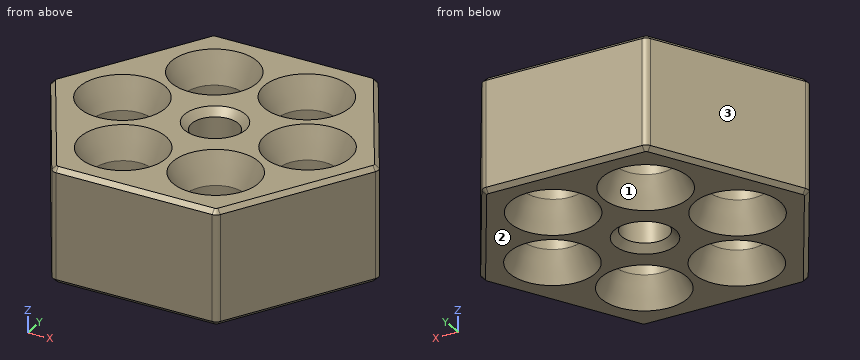
Autodesk Fusion 360 part; units mm, degrees
sketch "Sketch1" plane through (0, 0, 0) normal (0, 0, 1) x (1, 0, 0)
  line L0 (-5.7735, 10) -> (-11.547, 0)
  line L1 (-11.547, 0) -> (-5.7735, -10)
  line L2 (-5.7735, -10) -> (5.7735, -10)
  line L3 (5.7735, -10) -> (11.547, 0)
  line L4 (11.547, 0) -> (5.7735, 10)
  line L5 (5.7735, 10) -> (-5.7735, 10)
  circle A0 centre (0, 0) radius 1.625
  circle A1 centre (-3.25, 5.6292) radius 2.05
  line L6 (0, 0) -> (-5.7735, 10) construction
  circle A2 centre (-6.5, 0) radius 2.05
  circle A3 centre (-3.25, -5.6292) radius 2.05
  circle A4 centre (3.25, -5.6292) radius 2.05
  circle A5 centre (6.5, 0) radius 2.05
  circle A6 centre (3.25, 5.6292) radius 2.05
  circle A7 centre (0, 0) radius 6.5 construction
  dimension "d1" = 10
  dimension "d2" = 3.25
  dimension "d4" = 4.1
  dimension "d9" = 360
  dimension "d10" = 13
extrude "Extrude1" add sketch "Sketch1" along normal blind 8
chamfer "Chamfer3" distance 0.5 angle 45 1 edges at (-1.515, 0.5876, 0)
chamfer "Chamfer3" distance 0.5 angle 45 1 edges at (-1.515, 0.5876, 8)
fillet "Fillet1" radius 0.5 6 edges at (-5.7735, -10, 4) (5.7735, -10, 4) (11.547, 0, 4) (5.7735, 10, 4) (-5.7735, 10, 4) (-11.547, 0, 4)
chamfer "Chamfer4" distance 0.3 angle 45 24 edges at (0, -10, 8) (5.7348, -9.933, 8) (8.6603, -5, 8) (11.4697, 0, 8) (8.6603, 5, 8) (5.7348, 9.933, 8) (0, 10, 8) (-5.7348, 9.933, 8) (-8.6603, 5, 8) (-11.4697, 0, 8) (-8.6603, -5, 8) (-5.7348, -9.933, 8) (0, -10, 0) (5.7348, -9.933, 0) (8.6603, -5, 0) (11.4697, 0, 0) (8.6603, 5, 0) (5.7348, 9.933, 0) (0, 10, 0) (-5.7348, 9.933, 0) (-8.6603, 5, 0) (-11.4697, 0, 0) (-8.6603, -5, 0) (-5.7348, -9.933, 0)
chamfer "Chamfer2" distance 2 angle 25 6 edges at (1.3387, 6.3705, 8) (-5.1613, 6.3705, 8) (-8.4113, 0.7413, 8) (-5.1613, -4.8879, 8) (1.3387, -4.8879, 8) (4.5887, 0.7413, 8) measured on face at (5.2975, 5.527, 5.3333) measured on face at (-1.2025, 5.527, 5.3333) measured on face at (-4.4525, -0.1022, 5.3333) measured on face at (-1.2025, -5.7313, 5.3333) measured on face at (5.2975, -5.7313, 5.3333) measured on face at (8.5475, -0.1022, 5.3333)
chamfer "Chamfer5" distance 2 angle 25 6 edges at (-5.1613, -4.8879, 0) (1.3387, -4.8879, 0) (4.5887, 0.7413, 0) (1.3387, 6.3705, 0) (-5.1613, 6.3705, 0) (-8.4113, 0.7413, 0) measured on face at (-1.2102, -5.8333, 2) measured on face at (5.2898, -5.8333, 2) measured on face at (8.5398, -0.2041, 2) measured on face at (5.2898, 5.4251, 2) measured on face at (-1.2102, 5.4251, 2) measured on face at (-4.4602, -0.2041, 2)
CAD build for the part. Positions are in the model's coordinates, mm. Face numbers are marked on the shaded views. Round coordinates to 2 decimals unless told otherwise and drop trailing zeros. Write each loop counter-clockwise with the first axis right and the second up, starting at its lowest first coordinate (ties: lowest second). Pieces come first, ordered by that corner, then holes. Notation, with made-up numbers: (-19, 74.25) -> (35, 74.25) arc R24 ccw to (35, 111.25) -> close; hole circle Ø3 at (88, -40). An arc over 180 degrees is marked (long way). Answer as a JSON object with one key per item and string values.
(1) Band-saw the part on D-D, the plane y = -0.75. Count the separate pieces of the cut face and the enclosed holes in it, then the cut area to 3 significant figures.
Reported:
{"separate pieces": "4", "enclosed holes": "0", "area": "85.1 mm^2"}
(2) Two-plate mould, pull along X, no slides. Class the marked faces 1, 2 and 3: +X half, -X half, draft (parallel to the pull), parting line (faces both ways), or undercut.
Reported:
{"face 1": "undercut", "face 2": "draft", "face 3": "-X half"}
(3) Pin check, flat tips, straight feed: P1, Ø2, axis at y = -4, z = 4, coming from the -X side; P2, Ø5.5, axis at x = 6.5, y = 0, coming from the -Z side; P3, Ø1.5, axis at x = 6.5, z = 1.5, coming from the +Y side. Stop position of each tip, or through.
Reported:
{"P1": "stops at x = -9.81", "P2": "stops at z = 0.5", "P3": "stops at y = 9.92"}
(4) Band-saw the part on A-A, the plane x = 0. List the corners of the cut face in (y, z) (3 decimals), then the cut area to 3 significant figures.
Reported:
{"outline": "(-10, 0.3) -> (-9.7, 0) -> (-2.125, 0) -> (-1.625, 0.5) -> (-1.625, 7.5) -> (-2.125, 8) -> (-9.7, 8) -> (-10, 7.7) -> close; (1.625, 0.5) -> (2.125, 0) -> (9.7, 0) -> (10, 0.3) -> (10, 7.7) -> (9.7, 8) -> (2.125, 8) -> (1.625, 7.5) -> close", "area": "133 mm^2"}
(5) Band-saw the part on C-C, the plane x = 6.5. List the corners of the cut face in (y, z).
Reported:
{"outline": "(-8.74, 0.3) -> (-8.14, 0) -> (-2.98, 0) -> (-2.05, 2) -> (-2.05, 6) -> (-2.98, 8) -> (-8.14, 8) -> (-8.74, 7.7) -> close; (2.05, 2) -> (2.98, 0) -> (8.14, 0) -> (8.74, 0.3) -> (8.74, 7.7) -> (8.14, 8) -> (2.98, 8) -> (2.05, 6) -> close"}
(6) Band-saw the part on B-B, the plane x = 3.25. List the corners of the cut face in (y, z), then the cut area to 3 significant figures.
Reported:
{"outline": "(-10, 0.3) -> (-9.7, 0) -> (-8.61, 0) -> (-7.68, 2) -> (-7.68, 6) -> (-8.61, 8) -> (-9.7, 8) -> (-10, 7.7) -> close; (-3.58, 2) -> (-2.65, 0) -> (2.65, 0) -> (3.58, 2) -> (3.58, 6) -> (2.65, 8) -> (-2.65, 8) -> (-3.58, 6) -> close; (7.68, 2) -> (8.61, 0) -> (9.7, 0) -> (10, 0.3) -> (10, 7.7) -> (9.7, 8) -> (8.61, 8) -> (7.68, 6) -> close", "area": "86.8 mm^2"}
(7) Probe probe 1 along Y at (x, z) = (3.25, 3.7); probe 2 along Y at (x, z) = (-2.5, 3.25); probe 3 along X at (y, z) = (-6.25, 4.25). List the from-to ranges inside material, lowest first. Write a range as [from, to].
Reported:
{"probe 1": "y = [-10, -7.68], [-3.58, 3.58], [7.68, 10]", "probe 2": "y = [-10, -7.54], [-3.72, 3.72], [7.54, 10]", "probe 3": "x = [-7.94, -5.2], [-1.3, 1.3], [5.2, 7.94]"}
